```python
from build123d import *

# Parameters (mm, degrees)
SKETCH1_W           = 80
SKETCH1_H           = 39
SKETCH1_W_2         = 77
SKETCH1_H_2         = 36
BOSS_EXTRUDE1_DEPTH = 9
SKETCH2_W           = 80
SKETCH2_H           = 39
BOSS_EXTRUDE2_DEPTH = 1.5
SKETCH4_W           = 78.5
SKETCH4_H           = 37.5
CUT_EXTRUDE1_DEPTH  = 1
FILLET1_R           = 4
CUT_EXTRUDE2_REACH  = 58.844


with BuildPart() as part:
    # Sketch1 → Boss-Extrude1 (new body)
    with BuildSketch(Plane(origin=(0, 0, 0), x_dir=(1, 0, 0), z_dir=(0, 1, 0))):
        Rectangle(SKETCH1_W, SKETCH1_H)
        Rectangle(SKETCH1_W_2, SKETCH1_H_2, mode=Mode.SUBTRACT)
    extrude(amount=BOSS_EXTRUDE1_DEPTH)

    # Sketch2 → Boss-Extrude2 (add)
    with BuildSketch(Plane(origin=(0, 9, 0), x_dir=(1, 0, 0), z_dir=(0, 1, 0))):
        Rectangle(SKETCH2_W, SKETCH2_H)
    extrude(amount=BOSS_EXTRUDE2_DEPTH)

    # Sketch4 → Cut-Extrude1 (cut)
    with BuildSketch(Plane.XZ):
        Rectangle(SKETCH4_W, SKETCH4_H)
    extrude(amount=-CUT_EXTRUDE1_DEPTH, mode=Mode.SUBTRACT)

    # Fillet1
    fillet1_edges = [part.edges().sort_by_distance(p)[0] for p in [
        (-40, 10.5, 0),
        (0, 10.5, 19.5),
        (40, 10.5, 0),
        (0, 10.5, -19.5),
    ]]
    fillet(fillet1_edges, radius=FILLET1_R)

    # Sketch5 → Cut-Extrude2 (cut, up to next)
    with BuildSketch(Plane(origin=(0, 0, -19.5), x_dir=(-1, 0, 0), z_dir=(0, 0, -1)), mode=Mode.PRIVATE) as cut_extrude2_sk1:
        with BuildLine():
            Line((34.5, -3), (34.5, 3))
            ThreePointArc((34.5, 3), (36.5, 5), (38.5, 3))
            Line((38.5, 3), (38.5, -3))
            ThreePointArc((38.5, -3), (36.5, -5), (34.5, -3))
        make_face()
    cut_extrude2_tool1 = extrude(cut_extrude2_sk1.sketch, amount=-CUT_EXTRUDE2_REACH, mode=Mode.PRIVATE) & part.part
    add(cut_extrude2_tool1.solids().sort_by_distance((-36.5, 0, -19.5))[0], mode=Mode.SUBTRACT)


solid = part.part
```
Work out the finished part from the listing and answer in its coordinate system (mm). A direction names the side the tool comes from. Give positions to 0.01 mm unless a question says otherwise; leave off trailing zeros. Order: outer loops, then holes, each group sorted by start corner. A loop starts at its lowest first (then second) coordinate and runs counter-clockwise, first axis right, second up. Notation, with made-up numbers: M -16.5,86.25 L -5.5,86.25 A17 ccw -5.5,106.25 Z; hole C 23.5,-24.5 d1. An arc over 180 degrees is marked long. Return JSON: item names as keys, results as strings.
1) A tool of negligible diameter and unlimited length cuts with its end or side. For faces 5 (the cylindrical face through (-36.5, 5, -18.8)), 6 (the flat face through (-38.5, 5, -1)), 7 (the cylindrical face through (0.56, 9.359, 18.297)), from which of +Z, -Z, +X, -X, +Y, -Y can it reach the whole face along a straight path? Write none if from no direction.
Resolved:
{"face 5": "-Z, -Y", "face 6": "-Y", "face 7": "+Z, +X, -X, +Y"}
2) Each of these flat-tipped pins is pushed along its axis until it touches: pin 1 (1.5 mm diameter, centred on y = 9, z = -12, fed in from -X); pin 2 (11 mm diameter, centred on x = 8, z = -8.5, fed in from -Y). Where does it stop, or does it pass through?
Resolved:
{"pin 1": "x = -39.6", "pin 2": "y = 9"}
3) Section A-A, the plane z = 11 is taken. Write down the section's boundary in (x, y), plus the area to 3 significant figures.
Resolved:
{"outline": "M -40,0 L -39.25,0 L -39.25,1 L -38.5,1 L -38.5,9 L 38.5,9 L 38.5,1 L 39.25,1 L 39.25,0 L 40,0 L 40,6.5 A4 ccw 36,10.5 L -36,10.5 A4 ccw -40,6.5 Z", "area": "139 mm^2"}
4) Section C-C, the plane x = -22 is taken. Write down the section's boundary in (y, z), plus the area to 3 significant figures.
Resolved:
{"outline": "M 0,-19.5 L 6.5,-19.5 A4 ccw 10.5,-15.5 L 10.5,15.5 A4 ccw 6.5,19.5 L 0,19.5 L 0,18.75 L 1,18.75 L 1,18 L 9,18 L 9,-18 L 1,-18 L 1,-18.75 L 0,-18.75 Z", "area": "77.1 mm^2"}
5) Section D-D, the plane y = 7.25 is taken. Write down the section's boundary in (x, z), plus the area to 3 significant figures.
Resolved:
{"outline": "M -39.93,-19.43 L 39.93,-19.43 L 39.93,19.43 L -39.93,19.43 Z; hole M -38.5,-18 L 38.5,-18 L 38.5,18 L -38.5,18 Z", "area": "331 mm^2"}
6) Straight lines are drawn through the part: line 1 along X through (y, z) = (0.5, -13); line 2 along Z through (x, y) = (1, 2.75); line 3 along X through (y, z) = (5.25, -2). For each, find the intervals that lie inside material, in ascending order. Write a range as [from, to].
Resolved:
{"line 1": "[-40, -39.25], [39.25, 40]", "line 2": "[-19.5, -18], [18, 19.5]", "line 3": "[-40, -38.5], [38.5, 40]"}
7) For a pull along Z with two mould halves and no side action, classify faces 1 (the flat face through (-1, 9, 0)), 2 (the flat face through (38.5, 5, 0)), 3 (the cylindrical face through (-38.859, 9.297, -0.273)), 4 (the flat face through (-1, 3, -19.5)) as +Z half, -Z half, draft (parallel to the pull), parting line (faces both ways), or undercut.
Resolved:
{"face 1": "undercut", "face 2": "undercut", "face 3": "draft", "face 4": "-Z half"}
8) Section B-B, the plane y = 1.75 is taken. Write down the section's boundary in (x, z), plus the area to 3 significant figures.
Resolved:
{"outline": "M -40,-19.5 L -38.5,-19.5 L -38.5,18 L 38.5,18 L 38.5,-18 L -34.5,-18 L -34.5,-19.5 L 40,-19.5 L 40,19.5 L -40,19.5 Z", "area": "342 mm^2"}
